Part print with two shaded views. Sizes in mm from the minimum x, y, z corner. A direction names the side the tool comes from. Coordinates: 2 decimals unless noted, no trailing zeros. Loops run counter-clockwise (first coordinate to the right, second up) from the corner with the lowest first, then second, coordinate; pieces in that order, holes last.
Item 1: 3-axis set-ups, long thin cutter, end or side, ignore diameter. For the marked faces 4, 5, 6 and 7: which of +Z, -Z, +X, -X, +Y, -Y reach the whole face in a straight line?
Item 2: Cut at A-A (x = 20). List the corners of the cut face in (y, z).
Item 3: Cut at C-C (y = 1). List the corners of the cut face in (x, z), and give its area (3 significant figures).
Item 4: Mould opens along X. For the marked faces 1, 2 and 3 say: released by +X, released by -X, zero draft, split by the parting line, or undercut.
Item 5: Drill centre lines: line 1 along Z through (x, y) = (8.75, 7); line 2 along X through (y, z) = (5.75, 17.5); line 3 along X through (y, z) = (7.75, 15). Where is each one in solid material? Low to high.
Item 6: Cut at D-D (x = 8.75). List the corners of the cut face in (y, z), and give its area (3 significant figures).
Item 7: Flat gauge pins, fed straight in: pin 1 (2 mm diameter, centred on x = 16.5, y = 5.5, fed in from -Z); pin 2 (3 mm diameter, centred on x = 8.75, z = 3.75, fed in from -Y); pin 3 (6 mm diameter, centred on x = 10, z = 11, fed in from -Y); pin 4 (4 mm diameter, centred on y = 2, z = 32.5, fed in from -X). Where does each tip first touch, or does it go through?
Item 8: Cut at B-B (z = 3.75). List the corners of the cut face in (x, y), and give its area (3 significant figures).
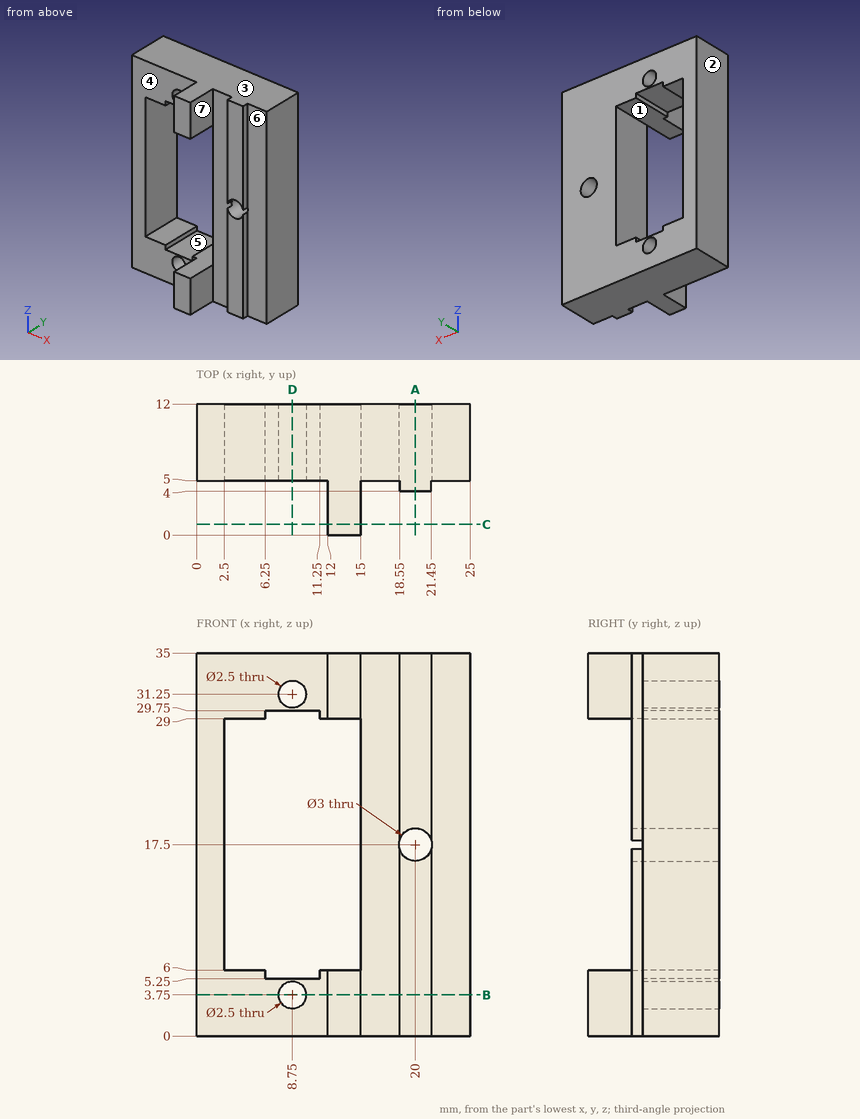
Filled sheet:
1. face 4: +Z, -Z, -X, -Y
1. face 5: +Y, -Y
1. face 6: +Z, -Z, +X, -Y
1. face 7: +Z, -Z, -Y
2. outline: (4, 0) - (12, 0) - (12, 16) - (4, 16) - close; (4, 19) - (12, 19) - (12, 35) - (4, 35) - close
3. outline: (12, 0) - (15, 0) - (15, 6) - (12, 6) - close; (12, 29) - (15, 29) - (15, 35) - (12, 35) - close
3. area: 36.0 mm2
4. face 1: undercut
4. face 2: released by -X
4. face 3: zero draft
5. line 1: z = 0 to 2.5, 5 to 5.25, 29.75 to 30, 32.5 to 35
5. line 2: x = 0 to 2.5, 15 to 18.5, 21.5 to 25
5. line 3: x = 0 to 2.5, 15 to 25
6. outline: (5, 0) - (12, 0) - (12, 2.5) - (5, 2.5) - close; (5, 5) - (12, 5) - (12, 5.25) - (5, 5.25) - close; (5, 29.75) - (12, 29.75) - (12, 30) - (5, 30) - close; (5, 32.5) - (12, 32.5) - (12, 35) - (5, 35) - close
6. area: 38.5 mm2
7. pin 1: stops at z = 0
7. pin 2: stops at y = 5
7. pin 3: passes through
7. pin 4: stops at x = 12
8. outline: (0, 5) - (7.5, 5) - (7.5, 12) - (0, 12) - close; (10, 5) - (12, 5) - (12, 0) - (15, 0) - (15, 5) - (18.55, 5) - (18.55, 4) - (21.45, 4) - (21.45, 5) - (25, 5) - (25, 12) - (10, 12) - close
8. area: 175 mm2
